CAD build for the part. Positions are in the model's coordinates, mm. Face numbers are marked on the shaded views. A direction names the side the tool comes from. Coordinates: 2 decimals unless noted, no trailing zeros. Order: outer loops, then holes, each group sorted by start corner. A loop starts at its lowest first (then second) coordinate and runs counter-clockwise, first axis right, second up. Notation, with made-up numbers: M 87,13 L 106,13 A21 cw 106,21 Z; hole C 30.5,68 d1. An arc over 180 degrees is marked long. One line per item, written item: value.
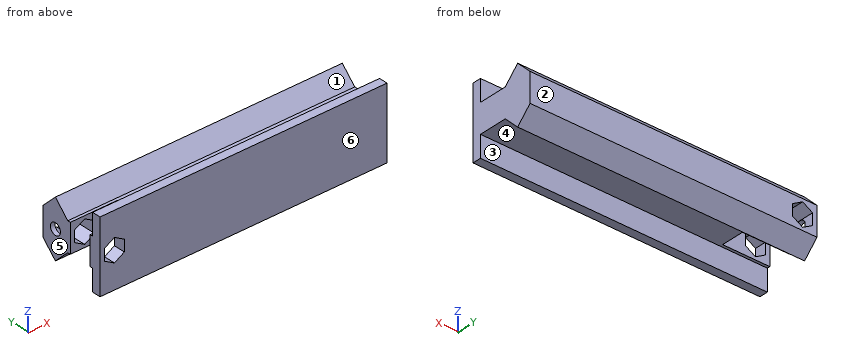
from build123d import *

# Parameters (mm, degrees)
BOSS_EXTRUDE1_DEPTH     = 50
SKETCH2_R               = 12.5
CUT_EXTRUDE1_DEPTH      = 4
CUT_EXTRUDE3_DEPTH      = 54.677276384
CUT_EXTRUDE3_DEPTH_BACK = 54.677276384
SKETCH6_R               = 2
CUT_EXTRUDE4_DEPTH      = 4


with BuildPart() as part:
    # Sketch1 → Boss-Extrude1 (new, symmetric)
    with BuildSketch(Plane(origin=(0, 0, 0), x_dir=(0, 0, -1), z_dir=(1, 0, 0))):
        Polygon((5, 5), (10, 10), (5, 15), (-5, 15), (-10, 10), (-5, 5), (-5, -5), (-12.5, -5), (-12.5, -8), (12.5, -8), (12.5, -5), (5, -5), align=None)
    extrude(amount=BOSS_EXTRUDE1_DEPTH, both=True)

    # Sketch2 → Cut-Extrude1 (cut, symmetric)
    with BuildSketch(Plane(origin=(0, 0, 0), x_dir=(1, 0, 0), z_dir=(0, 1, 0))):
        with Locations((-45, 0)):
            Circle(SKETCH2_R)
    extrude(amount=CUT_EXTRUDE1_DEPTH, both=True, mode=Mode.SUBTRACT)

    # Sketch4 → Cut-Extrude3 (cut, two sides: drawn at the far end of the back side and taken through both)
    with BuildSketch(Plane(origin=(0, 0, 0), x_dir=(1, 0, 0), z_dir=(0, 1, 0)).offset(-CUT_EXTRUDE3_DEPTH_BACK)):
        Polygon((-45, -4), (-41.535898385, -2), (-41.535898385, 2), (-45, 4), (-48.464101615, 2), (-48.464101615, -2), align=None)
    extrude(amount=CUT_EXTRUDE3_DEPTH + CUT_EXTRUDE3_DEPTH_BACK, mode=Mode.SUBTRACT)

    # Sketch6 → Cut-Extrude4 (cut)
    with BuildSketch(Plane.ZY.offset(50)):
        with Locations((0, 10)):
            Circle(SKETCH6_R)
    extrude(amount=-CUT_EXTRUDE4_DEPTH, mode=Mode.SUBTRACT)


solid = part.part
Q1. Slice it at A-A (z = 7.5). List the corners of the cut face in (x, y), plus the area to 3 significant figures.
Recorded:
outline: M -50,-8 L 50,-8 L 50,-5 L -50,-5 Z; M -50,7.5 L 50,7.5 L 50,12.5 L -50,12.5 Z
area: 800 mm^2
Q2. Slice it at C-C (y = -6). List the corners of the cut face in (x, z), plus the area to 3 significant figures.
Recorded:
outline: M -50,-12.5 L 50,-12.5 L 50,12.5 L -50,12.5 Z; hole M -48.46,-2 L -45,-4 L -41.54,-2 L -41.54,2 L -45,4 L -48.46,2 Z
area: 2,460 mm^2
Q3. Drill centre lines: line 1 along Y through (x, z) = (-49.55, 0); line 2 along X through (y, z) = (-4.25, 1); line 3 along Y through (x, z) = (14, 9.5). Where is each one in solid material? Low to high.
Recorded:
line 1: y = -8 to -4, 4 to 8, 12 to 15
line 2: x = -50 to -48.46, -41.54 to 50
line 3: y = -8 to -5, 9.5 to 10.5
Q4. Pin check, flat tips, straight feed: pin 1 Ø1.2 at (y, z) = (11, 0) entering from -X; pin 2 Ø6 at (x, y) = (29, 2.5) entering from -Z; pin 3 Ø4 at (x, z) = (15, -8.5) entering from +Y. Stop position of each tip, or through.
Recorded:
pin 1: stops at x = -41.54
pin 2: stops at z = -5.5
pin 3: stops at y = 13.5
Q5. Slice it at D-D (z = -9). List the corners of the cut face in (x, y).
Recorded:
outline: M -50,-8 L 50,-8 L 50,-5 L -50,-5 Z; M -50,9 L 50,9 L 50,11 L -50,11 Z
Q6. Mould opens along Y. For the marked faces 4, 5 and 6 say: released by +Y, released by -Y, zero draft, split by the parting line, or undercut.
Recorded:
face 4: undercut
face 5: zero draft
face 6: released by -Y
Q7. Which spindle directions (+Z, -Z, +X, -X, +Y, -Y) get a long thin tool onto all of the face, cutting with end or side? Do the marked faces 1, 2 and 3. Say none if no direction does.
Recorded:
face 1: +Z, +X, -X
face 2: +Z, -Z, +X, -X, +Y
face 3: -Z, +X, -X
Q8. Slice it at B-B (z = 0). List the corners of the cut face in (x, y), plus the area to 3 significant figures.
Recorded:
outline: M -50,-8 L -48.46,-8 L -48.46,-4 L -50,-4 Z; M -50,4 L -48.46,4 L -48.46,8 L -50,8 Z; M -50,12 L -48.46,12 L -48.46,15 L -50,15 Z; M -41.54,-8 L 50,-8 L 50,15 L -41.54,15 L -41.54,4 L -32.5,4 L -32.5,-4 L -41.54,-4 Z
area: 2,050 mm^2
